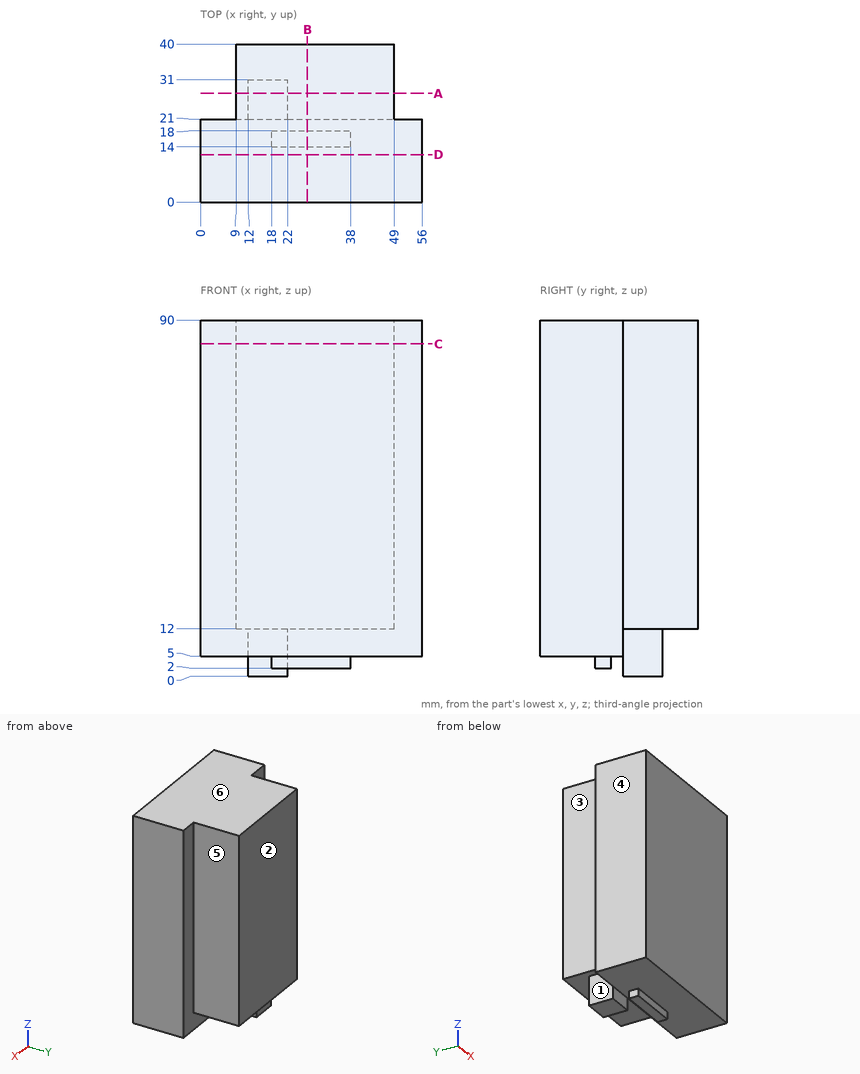
Source: three-view drawing plus pictorial views. Frame: mm from the lowest corner of the part. A direction names the side the tool comes from. Coordinates: 2 decimals unless noted, no trailing zeros. Write each loop counter-clockwise with the first axis right and the second up, starting at its lowest first coordinate (ties: lowest second). Pieces come first, ordered by that corner, then holes. Notation, with made-up numbers: (-33, 81) - (18, 81) arc R19 cw to (18, 118) - close; hole circle Ø5 at (-38.5, 25). An arc over 180 degrees is marked (long way). Return JSON: item names as keys, results as strings.
Item 1: Reachability of the marked faces 1, 2 and 3 from +Z, -Z, +X, -X, +Y, -Y: full face, straight path, thin tool, end or side. Return the list, or none.
Completed:
{"face 1": "-Z, -X, +Y", "face 2": "+Z, -Z, +X, -X, +Y", "face 3": "+Z, -Z, -X, +Y"}
Item 2: Pin query (flat end, axial travel): pin 1 Ø11 at (x, z) = (18, 5.5) entering from +Y; pin 2 Ø2 at (x, z) = (9, 63) entering from -Y; pin 3 Ø4 at (x, y) = (26.5, 14.5) entering from -Z; pin 4 Ø1.5 at (y, z) = (16.5, 3.5) entering from +X. Return the tip coordinate at first contact, or that it passes through.
Completed:
{"pin 1": "stops at y = 31", "pin 2": "stops at y = 0", "pin 3": "stops at z = 2", "pin 4": "stops at x = 38"}
Item 3: Line query: L1, parallel to Z at x = 51.5, y = 6; L2, parallel to X at y = 30.5, z = 77; L3, parallel to Y at x = 49.5, z = 68.5. Output: solid intervals per line, ascending.
Completed:
{"L1": "z = 5 to 90", "L2": "x = 9 to 49", "L3": "y = 0 to 21"}
Item 4: Section query A-A (y = 27.5). Output: boundary loops of the cut face in (x, z).
Completed:
{"outline": "(9, 12) - (12, 12) - (12, 0) - (22, 0) - (22, 12) - (49, 12) - (49, 90) - (9, 90) - close"}
Item 5: Section query B-B (x = 27). Output: boundary loops of the cut face in (y, z), and give its area (3 significant figures).
Completed:
{"outline": "(0, 5) - (14, 5) - (14, 2) - (18, 2) - (18, 5) - (21, 5) - (21, 12) - (40, 12) - (40, 90) - (0, 90) - close", "area": "3,280 mm2"}
Item 6: Section query C-C (z = 84). Output: boundary loops of the cut face in (x, y).
Completed:
{"outline": "(0, 0) - (56, 0) - (56, 21) - (49, 21) - (49, 40) - (9, 40) - (9, 21) - (0, 21) - close"}
Item 7: Section query D-D (y = 12). Output: boundary loops of the cut face in (x, z), and give its area (3 significant figures).
Completed:
{"outline": "(0, 5) - (56, 5) - (56, 90) - (0, 90) - close", "area": "4,760 mm2"}
Item 8: Pull-direction query (X, two-part tool) for the marked faces 4, 5 and 6; classes: +X half, -X half, draft (parallel to the pull), parting line (faces both ways), or undercut.
Completed:
{"face 4": "-X half", "face 5": "+X half", "face 6": "draft"}
